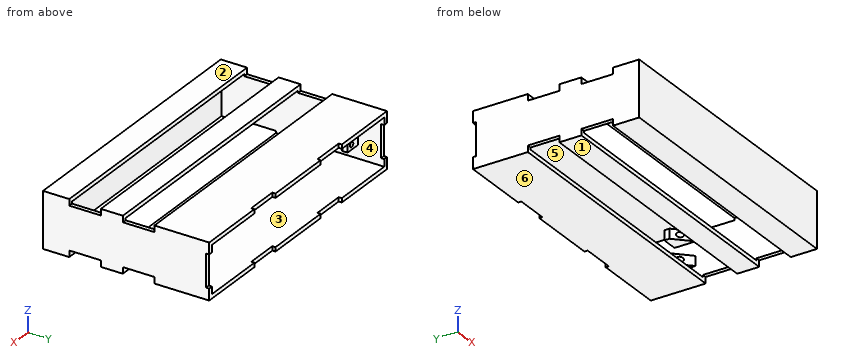
from build123d import *

# Parameters (mm, degrees)
SKETCH1_W                        = 261
SKETCH1_H                        = 52.8
BOSS_EXTRUDE1_DEPTH              = 3.175
SKETCH2_W                        = 261
SKETCH2_H                        = 52.8
SKETCH2_W_2                      = 253
SKETCH2_H_2                      = 44.8
BOSS_EXTRUDE2_DEPTH              = 155
SKETCH3_W                        = 6
SKETCH3_H                        = 30
CUT_EXTRUDE1_DEPTH               = 307.328729676
SKETCH4_W                        = 9.2
SKETCH4_H                        = 20
BOSS_EXTRUDE3_DEPTH              = 15
CHAMFER2_SIZE                    = 15
F_13_0_185_DIAMETER_HOLE1_REACH  = 190.192
F_13_0_185_DIAMETER_HOLE1_BORE_R = 2.3495
LPATTERN1_COUNT                  = 2
LPATTERN1_PITCH                  = 22.4
SKETCH7_W                        = 4
SKETCH7_H                        = 15.5
SKETCH7_W_2                      = 31
SKETCH7_H_2                      = 4
CUT_EXTRUDE2_DEPTH               = 3


# Read off the part's stored shape, not the designer's step: Mirror2
with BuildPart() as part:
    # Sketch1 → Boss-Extrude1 (new body)
    with BuildSketch(Plane(origin=(0, 0, 0), x_dir=(1, 0, 0), z_dir=(0, 1, 0))):
        Rectangle(SKETCH1_W, SKETCH1_H)
    extrude(amount=BOSS_EXTRUDE1_DEPTH)

    # Sketch2 → Boss-Extrude2 (add)
    with BuildSketch(Plane(origin=(0, 3.175, 0), x_dir=(1, 0, 0), z_dir=(0, 1, 0))):
        Rectangle(SKETCH2_W, SKETCH2_H)
        Rectangle(SKETCH2_W_2, SKETCH2_H_2, mode=Mode.SUBTRACT)
    extrude(amount=BOSS_EXTRUDE2_DEPTH)

    # Sketch3 → Cut-Extrude1 (cut, through all)
    with BuildSketch(Plane(origin=(130.5, 0, 0), x_dir=(0, 0, -1), z_dir=(1, 0, 0))):
        with Locations((-23.4, 91)):
            Rectangle(SKETCH3_W, SKETCH3_H)
        with Locations((-23.4, 40)):
            Rectangle(SKETCH3_W, SKETCH3_H)
    cut_extrude1 = extrude(amount=-CUT_EXTRUDE1_DEPTH, mode=Mode.SUBTRACT)

    # Mirror1: Cut-Extrude1 across plane
    add(cut_extrude1.mirror(Plane.XY), mode=Mode.SUBTRACT)

    # Sketch4 → Boss-Extrude3 (add)
    with BuildSketch(Plane.ZY.offset(-126.5)):
        with Locations((-5.6, 123)):
            Rectangle(SKETCH4_W, SKETCH4_H)
        with Locations((16.8, 123)):
            Rectangle(SKETCH4_W, SKETCH4_H)
    extrude(amount=BOSS_EXTRUDE3_DEPTH)

    # Chamfer2
    chamfer2_edges = [part.edges().sort_by_distance(p)[0] for p in [
        (111.5, 113, 16.8),
        (111.5, 113, -5.6),
    ]]
    chamfer(chamfer2_edges, length=CHAMFER2_SIZE - 0.0001)  # a hair under: the kernel refuses the full size

    # #13 (0.185) Diameter Hole1 bore → #13 (0.185) Diameter Hole1 (cut, up to next)
    with BuildSketch(Plane(origin=(0, 133, 0), x_dir=(1, 0, 0), z_dir=(0, 1, 0)), mode=Mode.PRIVATE) as f_13_0_185_diameter_hole1_sk1:
        with Locations((117.5, -16.8)):
            Circle(F_13_0_185_DIAMETER_HOLE1_BORE_R)
    f_13_0_185_diameter_hole1_tool1 = extrude(f_13_0_185_diameter_hole1_sk1.sketch, amount=-F_13_0_185_DIAMETER_HOLE1_REACH, mode=Mode.PRIVATE) & part.part
    f_13_0_185_diameter_hole1 = f_13_0_185_diameter_hole1_tool1.solids().sort_by_distance((117.5, 133, 16.8))[0]
    add(f_13_0_185_diameter_hole1, mode=Mode.SUBTRACT)

    # LPattern1: #13 (0.185) Diameter Hole1 ×2
    with Locations(*[(0, 0, -i * LPATTERN1_PITCH) for i in range(1, LPATTERN1_COUNT)]):
        add(f_13_0_185_diameter_hole1, mode=Mode.SUBTRACT)

    # Mirror2: part across plane


with BuildPart() as part_1:
    add(part.part)
    add(part.part.mirror(Plane(origin=(0, 0, 0), x_dir=(0, 0, 1), z_dir=(1, 0, 0))))

    # Sketch7 → Cut-Extrude2 (cut)
    with BuildSketch(Plane(origin=(0, 158.175, 0), x_dir=(1, 0, 0), z_dir=(0, 1, 0))):
        with Locations((128.5, 7.75)):
            Rectangle(SKETCH7_W, SKETCH7_H)
        with Locations((48.666666667, 24.4)):
            Rectangle(SKETCH7_W_2, SKETCH7_H_2)
        with Locations((-128.5, 7.75)):
            Rectangle(SKETCH7_W, SKETCH7_H)
        with Locations((-48.666666667, 24.4)):
            Rectangle(SKETCH7_W_2, SKETCH7_H_2)
    cut_extrude2 = extrude(amount=-CUT_EXTRUDE2_DEPTH, mode=Mode.SUBTRACT)

    # Mirror3: Cut-Extrude2 across plane
    add(cut_extrude2.mirror(Plane.XY), mode=Mode.SUBTRACT)


solid = part_1.part
The listing builds one solid part. Answer for the finished solid, in the listing's coordinates (mm). Face numbers are marked on the shaded views. A direction names the side the tool comes from. Round coordinates to 2 decimals unless told otherwise and drop trailing zeros. Order: outer loops, then holes, each group sorted by start corner. A loop starts at its lowest first (then second) coordinate and runs counter-clockwise, first axis right, second up. Notation, with made-up numbers: (78, 35.25) -> (127, 35.25) arc R8 cw to (127, 42.25) -> close; hole circle Ø11 at (-36, 17). An arc over 180 degrees is marked (long way). Write each question's results on one line, items separated by ' | '. Start each with the question number.
Q1. Find section A-A (x = 56). Determine the outline of the cut face in (y, z) (3 decimals), then the cut area to 3 significant figures.
Q2. Find section C-C (y = 21). Determine the outline of the cut face in (x, z), then the cut area to 3 significant figures.
Q3. Which of the six approach directions +Z, -Z, +X, -X, +Y, -Y give full straight-line access (tool end or side, diameter ignored) to the marked faces 4, 5 and 6?
Q4. Each of these flat-tipped pins is pushed along its axis until it touches: pin 1 (6.5 mm diameter, centred on x = 33.5, z = -23.5, fed in from +Y) (3 decimals); pin 2 (3 mm diameter, centred on x = 129, z = -2.5, fed in from +Y) (3 decimals); pin 3 (5.5 mm diameter, centred on x = -117.5, z = 16.8, fed in from +Y). Where does it stop, or does it pass through?
Q5. Find section B-B (y = 96). Determine the outline of the cut face in (x, z), then the cut area to 3 significant figures.
Q6. The mould has two halves that part along Z. Classify the marked faces 1, 2 and 3: pulls with the +Z half, pulls with the -Z half, needs draft (parallel to the pull), parting line crosses it, or undercut.
Q7. Straight lines are drawn through the part: probe 1 along X at (y, z) = (128, 16.8); probe 2 along Y at (x, z) = (10.5, 22.5) (3 decimals); probe 3 along Z at (x, y) = (-117.5, 126.5). For each, find the intervals that lie inside material, in ascending order. Write a range as from..to.
Q8. Find section D-D (x = 18). Determine the outline of the cut face in (y, z) (3 decimals), then the cut area to 3 significant figures.
Worked answers:
1) outline: (0, -26.4) -> (25, -26.4) -> (25, -22.4) -> (3.175, -22.4) -> (3.175, 22.4) -> (25, 22.4) -> (25, 26.4) -> (0, 26.4) -> close; (55, -26.4) -> (76, -26.4) -> (76, -22.4) -> (55, -22.4) -> close; (55, 22.4) -> (76, 22.4) -> (76, 26.4) -> (55, 26.4) -> close; (106, -26.4) -> (155.175, -26.4) -> (155.175, -22.4) -> (106, -22.4) -> close; (106, 22.4) -> (155.175, 22.4) -> (155.175, 26.4) -> (106, 26.4) -> close | area: 904 mm2
2) outline: (-130.5, -26.4) -> (130.5, -26.4) -> (130.5, 26.4) -> (-130.5, 26.4) -> close; hole (-126.5, -22.4) -> (126.5, -22.4) -> (126.5, 22.4) -> (-126.5, 22.4) -> close | area: 2,450 mm2
3) face 4: none | face 5: +Y | face 6: -Z, +X, -X, +Y, -Y
4) pin 1: stops at y = 158.175 | pin 2: stops at y = 155.175 | pin 3: stops at y = 133
5) outline: (-130.5, -20.4) -> (-126.5, -20.4) -> (-126.5, 20.4) -> (-130.5, 20.4) -> close; (126.5, -20.4) -> (130.5, -20.4) -> (130.5, 20.4) -> (126.5, 20.4) -> close | area: 326 mm2
6) face 1: pulls with the -Z half | face 2: pulls with the +Z half | face 3: undercut
7) probe 1: x = -130.5..-119.85, -115.15..-111.5, 111.5..115.15, 119.85..130.5 | probe 2: y = 0..25, 55..76, 106..158.175 | probe 3: z = -26.4..-22.4, -10.2..-7.95, -3.25..-1, 12.2..14.45, 19.15..21.4, 22.4..26.4
8) outline: (0, -26.4) -> (25, -26.4) -> (25, -22.4) -> (3.175, -22.4) -> (3.175, 22.4) -> (25, 22.4) -> (25, 26.4) -> (0, 26.4) -> close; (55, -26.4) -> (76, -26.4) -> (76, -22.4) -> (55, -22.4) -> close; (55, 22.4) -> (76, 22.4) -> (76, 26.4) -> (55, 26.4) -> close; (106, -26.4) -> (158.175, -26.4) -> (158.175, -22.4) -> (106, -22.4) -> close; (106, 22.4) -> (158.175, 22.4) -> (158.175, 26.4) -> (106, 26.4) -> close | area: 928 mm2
